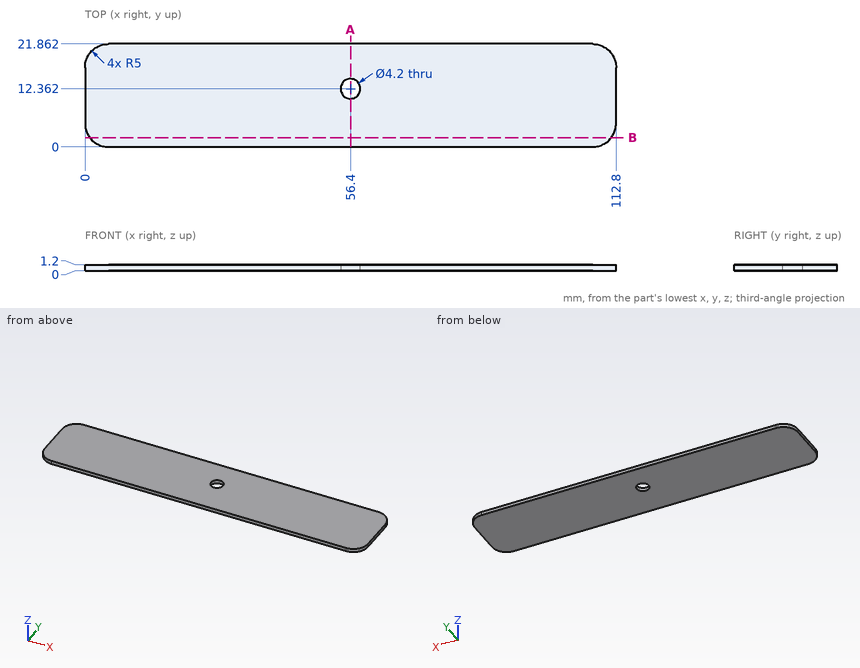
For this review, use the dimensioned drawing (mm, ordinates from the lowest corner) and the shaded views. Round coordinates to 2 decimals unless told otherwise and drop trailing zeros. Write each loop counter-clockwise with the first axis right and the second up, starting at its lowest first coordinate (ties: lowest second). Pieces come first, ordered by that corner, then holes. Notation, with made-up numbers: (64.5, 3) -> (120.5, 3) arc R14 ccw to (120.5, 13) -> close; hole circle Ø10 at (83, 6). An arc over 180 degrees is marked (long way). Answer in a Markdown table with one row per item.
Q1. Clearance check with a flat-ended pin moving along its axis: pin 1 Ø4 at (x, y) = (56.4, 12.36) entering from +Z. State where the tip first meets the part, or that it passes through.
The answers:
| item | result |
|---|---|
| pin 1 | through |
Q2. Take a section at A-A, the plane x = 56.4. State the section outline as (y, z) points.
The answers:
| item | result |
|---|---|
| outline | (0, 0) -> (10.26, 0) -> (10.26, 1.2) -> (0, 1.2) -> close; (14.46, 0) -> (21.86, 0) -> (21.86, 1.2) -> (14.46, 1.2) -> close |
Q3. To check wall thickness, follow L1, parallel to Y at x = 56.4, z = 0.3; L2, parallel to Y at x = 108, z = 0.55; L3, parallel to X at y = 10.5, z = 0.75 (1 decimal). State the ranges of each line that lie inside material, in increasing order. Write a range as [from, to].
The answers:
| item | result |
|---|---|
| L1 | [0, 10.26], [14.46, 21.86] |
| L2 | [0, 21.86] |
| L3 | [0, 55.4], [57.4, 112.8] |
Q4. Take a section at B-B, the plane y = 2. State the section outline as (x, z) points.
The answers:
| item | result |
|---|---|
| outline | (1, 0) -> (111.8, 0) -> (111.8, 1.2) -> (1, 1.2) -> close |
